Can you work these out from the drawing? Everything is in mm from the part's minimum corner. Round coordinates to 2 decimals unless told otherwise and drop trailing zeros. Order: outer loops, then holes, each group sorted by start corner. A loop starts at its lowest first (then second) coordinate and runs counter-clockwise, first axis right, second up. Notation, with made-up numbers: M 37.25,26.5 L 53.25,26.5 A11 cw 53.25,30.5 Z; hole C 18,-21 d2. An arc over 180 degrees is marked long. Answer as a JSON object with one key per item and string values. Group by question number.
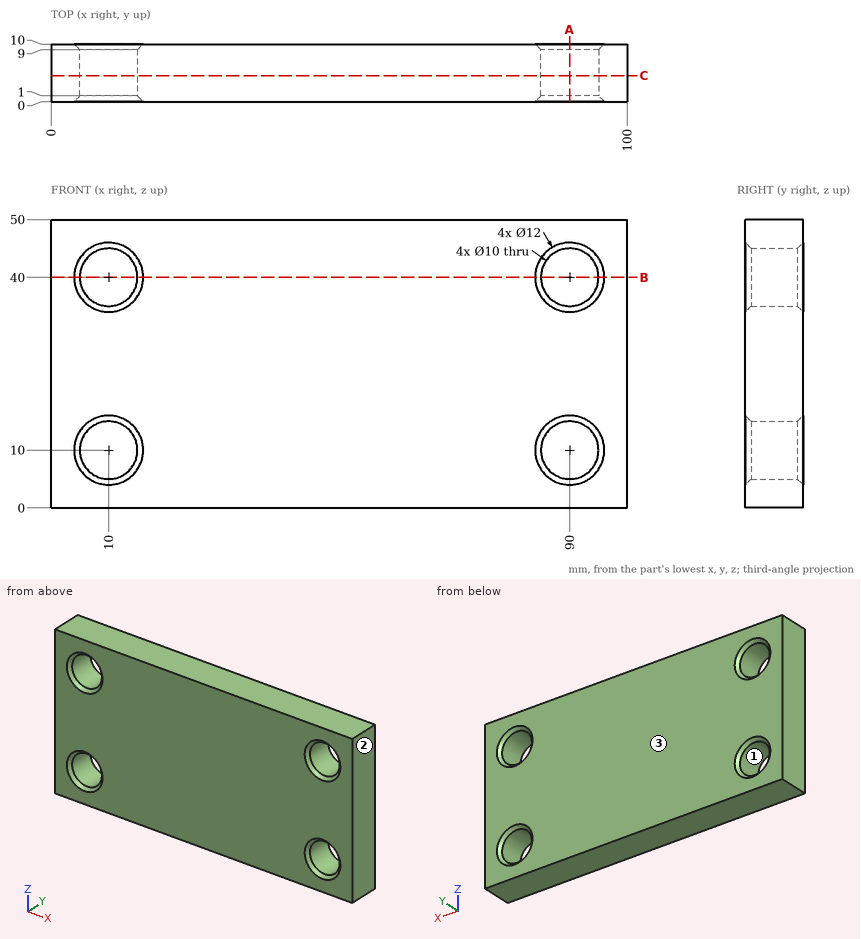
Item 1: Suppose I cut it at B-B, the plane z = 40. Write out the boundary of the cut face in (x, y), and give its area (3 significant figures).
Item 2: I'm going to push a flat-ended pin straight in: pin 1 Ø11.5 at (x, z) = (90, 10) entering from -Y. Where does the tip first touch, or does it pass through?
Item 3: Suppose I cut it at C-C, the plane y = 4.5. Write out the boundary of the cut face in (x, z).
Item 4: If we mould it in two halves opening along X, with no side actions, what happens to the marked faces 1, 2 and 3? For each: +X half, -X half, draft (parallel to the pull), parting line (faces both ways), or undercut.
Item 5: Suppose I cut it at A-A, the plane x = 90. Write out the boundary of the cut face in (y, z), and give its area (3 significant figures).
Item 6: I need wall thicknesses on line 1 (Z direction, x = 90, y = 4.5); line 2 (Z direction, x = 14, y = 7); line 3 (X direction, y = 1.5, z = 38.5). Which ranges of each line are inside material? Lowest first, please.
Computed:
{
 "1": {"outline": "M 0,0 L 4,0 L 5,1 L 5,9 L 4,10 L 0,10 Z; M 15,1 L 16,0 L 84,0 L 85,1 L 85,9 L 84,10 L 16,10 L 15,9 Z; M 95,1 L 96,0 L 100,0 L 100,10 L 96,10 L 95,9 Z", "area": "796 mm^2"},
 "2": {"pin 1": "stops at y = 0.25"},
 "3": {"outline": "M 0,0 L 100,0 L 100,50 L 0,50 Z; hole C 10,10 d10; hole C 10,40 d10; hole C 90,10 d10; hole C 90,40 d10"},
 "4": {"face 1": "undercut", "face 2": "+X half", "face 3": "draft"},
 "5": {"outline": "M 0,0 L 10,0 L 10,4 L 9,5 L 1,5 L 0,4 Z; M 0,16 L 1,15 L 9,15 L 10,16 L 10,34 L 9,35 L 1,35 L 0,34 Z; M 0,46 L 1,45 L 9,45 L 10,46 L 10,50 L 0,50 Z", "area": "296 mm^2"},
 "6": {"line 1": "z = 0 to 5, 15 to 35, 45 to 50", "line 2": "z = 0 to 7, 13 to 37, 43 to 50", "line 3": "x = 0 to 5.23, 14.77 to 85.23, 94.77 to 100"}
}
